from build123d import *

# Parameters (mm, degrees)
SKETCH_1_R      = 1.75
SKETCH_1_R_2    = 6.75
SKETCH_1_R_3    = 2.50825
EXTRUDE_1_DEPTH = 3.175


with BuildPart() as part:
    # Эскиз1 → Бобышка-Вытянуть1 (new body)
    with BuildSketch(Plane.XY):
        Polygon((22.225, 86.36), (-22.225, 86.36), (-22.225, 35.56), (-22.225, 0), (22.225, 0), (22.225, 35.56), align=None)
        with Locations((-7.75, 63.353393759)):
            Circle(SKETCH_1_R, mode=Mode.SUBTRACT)
        with Locations((-15.5, 49.93)):
            Circle(SKETCH_1_R, mode=Mode.SUBTRACT)
        with Locations((-7.75, 36.506606241)):
            Circle(SKETCH_1_R, mode=Mode.SUBTRACT)
        with Locations((7.75, 36.506606241)):
            Circle(SKETCH_1_R, mode=Mode.SUBTRACT)
        with Locations((15.5, 49.93)):
            Circle(SKETCH_1_R, mode=Mode.SUBTRACT)
        with Locations((7.75, 63.353393759)):
            Circle(SKETCH_1_R, mode=Mode.SUBTRACT)
        with Locations((0, 43.18)):
            Circle(SKETCH_1_R_2, mode=Mode.SUBTRACT)
        with Locations((15.875, 81.28)):
            Circle(SKETCH_1_R_3, mode=Mode.SUBTRACT)
        with Locations((-15.875, 81.28)):
            Circle(SKETCH_1_R_3, mode=Mode.SUBTRACT)
        with Locations((15.875, 5.08)):
            Circle(SKETCH_1_R_3, mode=Mode.SUBTRACT)
        with Locations((-15.875, 5.08)):
            Circle(SKETCH_1_R_3, mode=Mode.SUBTRACT)
    extrude(amount=EXTRUDE_1_DEPTH)


solid = part.part
The model under review builds one solid part; all positions refer to its coordinate system, in mm. Round coordinates to 2 decimals unless told otherwise and drop trailing zeros. Loops run counter-clockwise (first coordinate to the right, second up) from the corner with the lowest first, then second, coordinate; pieces in that order, holes last. Notation, with made-up numbers: M 2,-28.75 L 34,-28.75 A17 ccw 34,-21.75 Z; hole C 50.25,50.5 d10. An arc over 180 degrees is marked long. Answer as CSV lines item,"result".
1. We need section D-D (y = 81.28). Give the boundary of the cut face in (x, z) (3 decimals).
Outcome:
outline,"M -22.225,0 L -18.383,0 L -18.383,3.175 L -22.225,3.175 Z; M -13.367,0 L 13.367,0 L 13.367,3.175 L -13.367,3.175 Z; M 18.383,0 L 22.225,0 L 22.225,3.175 L 18.383,3.175 Z"
2. We need section B-B (y = 43.18). Give the boundary of the cut face in (x, z) (3 decimals), plus the area to 3 significant figures.
Outcome:
outline,"M -22.225,0 L -6.75,0 L -6.75,3.175 L -22.225,3.175 Z; M 6.75,0 L 22.225,0 L 22.225,3.175 L 6.75,3.175 Z"
area,"98.3 mm2"
3. To check wall thickness, follow L1, parallel to Y at x = -7.5, z = 2.15; L2, parallel to Y at x = -7.75, z = 1.8; L3, parallel to X at y = 81, z = 1.3 (3 decimals). State the ranges of each line that lie inside material, in increasing order. Write a range as [from, to].
Outcome:
L1,"y = [0, 34.77], [38.24, 61.62], [65.09, 86.36]"
L2,"y = [0, 34.76], [38.26, 61.6], [65.1, 86.36]"
L3,"x = [-22.225, -18.368], [-13.382, 13.382], [18.368, 22.225]"
4. Draft analysis for pull direction X (two halves, no side actions). For faces 1 (the face through (-22.225, 44, 2)), 2 (the face through (0, 0, 2)), 3 (the face through (22.225, 43, 2)), 4 (the face through (-6.94, 61.8, 1.57)), state which applies: pulls with the +X half, pulls with the -X half, needs draft (parallel to the pull), parting line crosses it, or undercut.
Outcome:
face 1,"pulls with the -X half"
face 2,"needs draft"
face 3,"pulls with the +X half"
face 4,"undercut"
5. We need section A-A (x = 0). Give the boundary of the cut face in (y, z) (3 decimals).
Outcome:
outline,"M 0,0 L 36.43,0 L 36.43,3.175 L 0,3.175 Z; M 49.93,0 L 86.36,0 L 86.36,3.175 L 49.93,3.175 Z"
6. Insertion check: pin 1 Ø4.5 at (x, y) = (15.875, 5.08) entering from +Z (3 decimals). The pin has a flat end and moves straight along its axis. Give the tip position at first contact, or say it passes through.
Outcome:
pin 1,"passes through"
7. We need section C-C (x = -7.75). Give the boundary of the cut face in (y, z) (3 decimals), plus the area to 3 significant figures.
Outcome:
outline,"M 0,0 L 34.757,0 L 34.757,3.175 L 0,3.175 Z; M 38.257,0 L 61.603,0 L 61.603,3.175 L 38.257,3.175 Z; M 65.103,0 L 86.36,0 L 86.36,3.175 L 65.103,3.175 Z"
area,"252 mm2"
